Autodesk Inventor part; units mm, degrees
ref_plane "YZ Plane" through (0, 0, 0) normal (1, 0, 0) x (0, 1, 0)
ref_plane "XZ Plane" through (0, 0, 0) normal (0, 1, 0) x (-1, 0, 0)
ref_plane "XY Plane" through (0, 0, 0) normal (0, 0, 1) x (1, 0, 0)
sketch "Sketch1" plane through (0, 0, 0) normal (0, 0, 1) x (1, 0, 0)
  line L0 (-55, 65) -> (55, 65)
  line L1 (55, 65) -> (55, -65)
  line L2 (55, -65) -> (-55, -65)
  line L3 (-55, -65) -> (-55, 65)
  point P0 (0, 0)
  dimension "d0" = 110
  dimension "d1" = 130
  dimension "d2" = 65
  dimension "d3" = 55
extrude "profile" add sketch "Sketch1" along normal blind 2.6568
sketch "Sketch3" plane through (0, 0, 2.6568) normal (0, 0, 1) x (1, 0, 0)
  line L0 (-55, 65) -> (-55, -65)
  line L1 (-55, -65) -> (55, -65)
  circle A0 centre (-43, -55) radius 3.57
  circle A1 centre (-43, 9.6) radius 2.75
  circle A2 centre (-43, 9.6) radius 11.75 construction
  point P0 (0, 0)
  dimension "d15" = 7.14
  dimension "d16" = 5.5
  dimension "d17" = 64.6
  dimension "d18" = 10
  dimension "d19" = 12
  dimension "d21" = 12
extrude "Extrusion3" cut sketch "Sketch3" against normal through all
pattern_linear "Rectangular Pattern2" count 2 spacing 88 along (1, 0, 0) of "Extrusion3"
sketch "Sketch4" plane through (0, 0, 2.6568) normal (0, 0, 1) x (1, 0, 0)
  line L0 (55, 65) -> (-55, 65)
  line L1 (55, -65) -> (55, 65)
  circle A0 centre (0, 36) radius 11.5
  circle A1 centre (-15.5, 51.5) radius 2
  circle A2 centre (15.5, 51.5) radius 2
  circle A3 centre (-15.5, 20.5) radius 2
  circle A4 centre (15.5, 20.5) radius 2
  point P0 (0, 0)
  dimension "d27" = 23
  dimension "d28" = 29
  dimension "d29" = 4
  dimension "d30" = 15.5
  dimension "d31" = 15.5
  dimension "d36" = 55
  dimension "d51" = 31
  dimension "d54" = 31
extrude "nema17_mount" cut sketch "Sketch4" against normal through all
fillet "Fillet1" radius 25 2 edges at (55, 65, 1.3284) (-55, 65, 1.3284)
sketch "Sketch5" plane through (0, 0, 2.6568) normal (0, 0, 1) x (1, 0, 0)
  line L0 (-55, 65) -> (-55, -65)
  line L1 (-55, -65) -> (55, -65)
  circle A0 centre (-10, 9.5) radius 2.75
  line L2 (30, 65) -> (-30, 65)
  circle A1 centre (10, 9.5) radius 2.75
  point P0 (67.5, -65)
  point P1 (-72.5, 60)
  point P2 (-72.5, -60)
  point P3 (-67.5, -65)
  point P4 (0, 0)
  dimension "d41" = 5.5
  dimension "d42" = 74.5
  dimension "d43" = 45
  dimension "d59" = 20
extrude "idler_holes" cut sketch "Sketch5" against normal through all
sketch "Sketch7" plane through (0, 0, 2.6568) normal (0, 0, 1) x (1, 0, 0)
  circle A0 centre (-15.5, 51.5) radius 2
  line L0 (-55, 40) -> (-55, -65)
  line L1 (30, 65) -> (-30, 65)
  arc A1 (-9.3427, 52.3297) -> (-11.7335, 57.1348) centre (-10, 55) ccw
  arc A2 (11.7395, 57.13) -> (8.8336, 52.5096) centre (10, 55) ccw
  line L2 (-11.7335, 57.1348) -> (-16.7607, 53.0526)
  line L3 (-8.2665, 52.8652) -> (-14.6091, 49.7094)
  circle A3 centre (15.5, 51.5) radius 2
  line L4 (8.8336, 52.5096) -> (14.6274, 49.7004)
  line L5 (16.9616, 52.8652) -> (11.7395, 57.13)
  point P0 (0, 0)
  dimension "d70" = 5.5
  dimension "d71" = 5.5
  dimension "d72" = 10
  dimension "d73" = 10
  dimension "d74" = 20
  dimension "d75" = 45
extrude "Extrusion7" cut sketch "Sketch7" against normal through all contours A0 L2 A1 L3 | L5 A3 L4 A2 | L5 A3 picked at (16.0496, 50.6933)
sketch "Sketch8" plane through (0, 0, 2.6568) normal (0, 0, 1) x (1, 0, 0)
  line L0 (-55, 40) -> (-55, -65)
  line L1 (-55, -65) -> (55, -65)
  circle A0 centre (-10, -55) radius 2.75
  circle A1 centre (10, -55) radius 2.75
  point P0 (0, 0)
  dimension "d78" = 5.5
  dimension "d79" = 5.5
  dimension "d80" = 20
  dimension "d81" = 10
  dimension "d82" = 10
  dimension "d83" = 45
extrude "Extrusion8" cut sketch "Sketch8" against normal through all
sketch "Sketch9" plane through (0, 0, 2.6568) normal (0, 0, 1) x (1, 0, 0)
  line L0 (-55, 40) -> (-55, -65)
  line L1 (-55, -65) -> (55, -65)
  circle A0 centre (-27.5, 7) radius 2.75
  point P0 (0, 0)
  dimension "d86" = 5.5
  dimension "d87" = 27.5
  dimension "d88" = 72
extrude "Extrusion9" cut sketch "Sketch9" against normal through all
pattern_linear "Rectangular Pattern4" count 2 spacing 55 along (1, 0, 0) count 2 spacing 62 along (0, -1, 0) of "Extrusion9"
fillet "Fillet3" radius 5 2 edges at (55, -65, 1.3284) (-55, -65, 1.3284)
sketch "Sketch10" plane through (0, 0, 2.6568) normal (0, 0, 1) x (1, 0, 0)
  line L0 (30, 65) -> (-30, 65)
  line L1 (-55, 40) -> (-55, -60)
  circle A0 centre (-27.5, 55) radius 2.75
  circle A1 centre (27.5, 55) radius 2.75
  point P0 (0, 0)
  dimension "d98" = 5.5
  dimension "d99" = 5.5
  dimension "d100" = 27.5
  dimension "d101" = 82.5
  dimension "d102" = 10
  dimension "d103" = 10
extrude "Extrusion10" cut sketch "Sketch10" against normal through all
equation "\"d72\" = d73"
equation "\"d82\" = d81"
properties part number "x_motor_mount_v2" material "Steel, Mild"
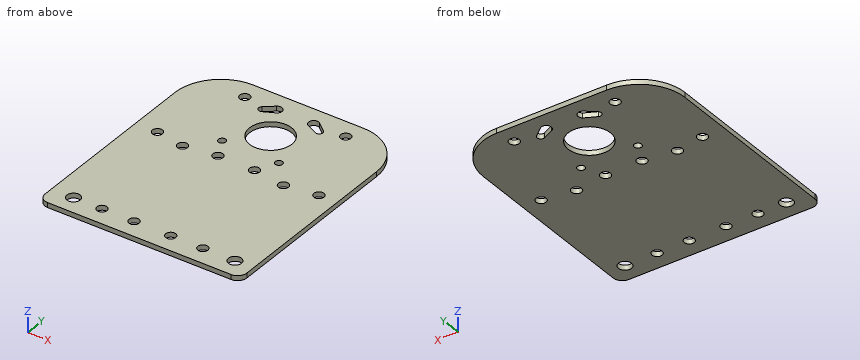
Read the model definition and answer for the solid it produces. Units are mm, in the model's axes. Give positions to 0.01 mm unless a question says otherwise; leave off trailing zeros. Write each loop counter-clockwise with the first axis right and the second up, starting at its lowest first coordinate (ties: lowest second). Pieces come first, ordered by that corner, then holes. Notation, with made-up numbers: (47.25, 73) - (77.25, 73) arc R19 cw to (77.25, 84) - close; hole circle Ø11 at (28, 27.25). An arc over 180 degrees is marked (long way). Use CSV: the item, a comma, the result in double quotes. Start each with the question number.
(1) Find section C-C (y = 20.5). Give the vertices of the cut face in (x, z), plus the area to 3 significant figures.
(2) Consider line 1 along Y through (x, z) = (-27.5, 0.95); line 2 along Y through (x, z) = (45, 1.75); line 3 along Y through (x, z) = (-10, 0.7). Determine where each line is inside the solid, lowest interval first.
(3) Find section A-A (x = 45). Give the vertices of the cut face in (y, z), plus the area to 3 significant figures.
(4) Find section D-D (x = 0). Give the vertices of the cut face in (y, z).
(5) Find section B-B (y = -55). Give the vertices of the cut face in (x, z), plus the area to 3 significant figures.
Findings below:
1,outline,"(-55, 0) - (-17.5, 0) - (-17.5, 2.66) - (-55, 2.66) - close; (-13.5, 0) - (13.5, 0) - (13.5, 2.66) - (-13.5, 2.66) - close; (17.5, 0) - (55, 0) - (55, 2.66) - (17.5, 2.66) - close"
1,area,"271 mm2"
2,line 1,"-65 to -57.75, -52.25 to 4.25, 9.75 to 52.25, 57.75 to 65"
2,line 2,"-65 to -58.57, -51.43 to 6.85, 12.35 to 60"
2,line 3,"-65 to -57.75, -52.25 to 6.75, 12.25 to 30.32, 41.68 to 52, 57.75 to 65"
3,outline,"(-65, 0) - (-58.57, 0) - (-58.57, 2.66) - (-65, 2.66) - close; (-51.43, 0) - (6.85, 0) - (6.85, 2.66) - (-51.43, 2.66) - close; (12.35, 0) - (60, 0) - (60, 2.66) - (12.35, 2.66) - close"
3,area,"299 mm2"
4,outline,"(-65, 0) - (24.5, 0) - (24.5, 2.66) - (-65, 2.66) - close; (47.5, 0) - (65, 0) - (65, 2.66) - (47.5, 2.66) - close"
5,outline,"(-55, 0) - (-46.57, 0) - (-46.57, 2.66) - (-55, 2.66) - close; (-39.43, 0) - (-30.25, 0) - (-30.25, 2.66) - (-39.43, 2.66) - close; (-24.75, 0) - (-12.75, 0) - (-12.75, 2.66) - (-24.75, 2.66) - close; (-7.25, 0) - (7.25, 0) - (7.25, 2.66) - (-7.25, 2.66) - close; (12.75, 0) - (24.75, 0) - (24.75, 2.66) - (12.75, 2.66) - close; (30.25, 0) - (41.43, 0) - (41.43, 2.66) - (30.25, 2.66) - close; (48.57, 0) - (55, 0) - (55, 2.66) - (48.57, 2.66) - close"
5,area,"196 mm2"
